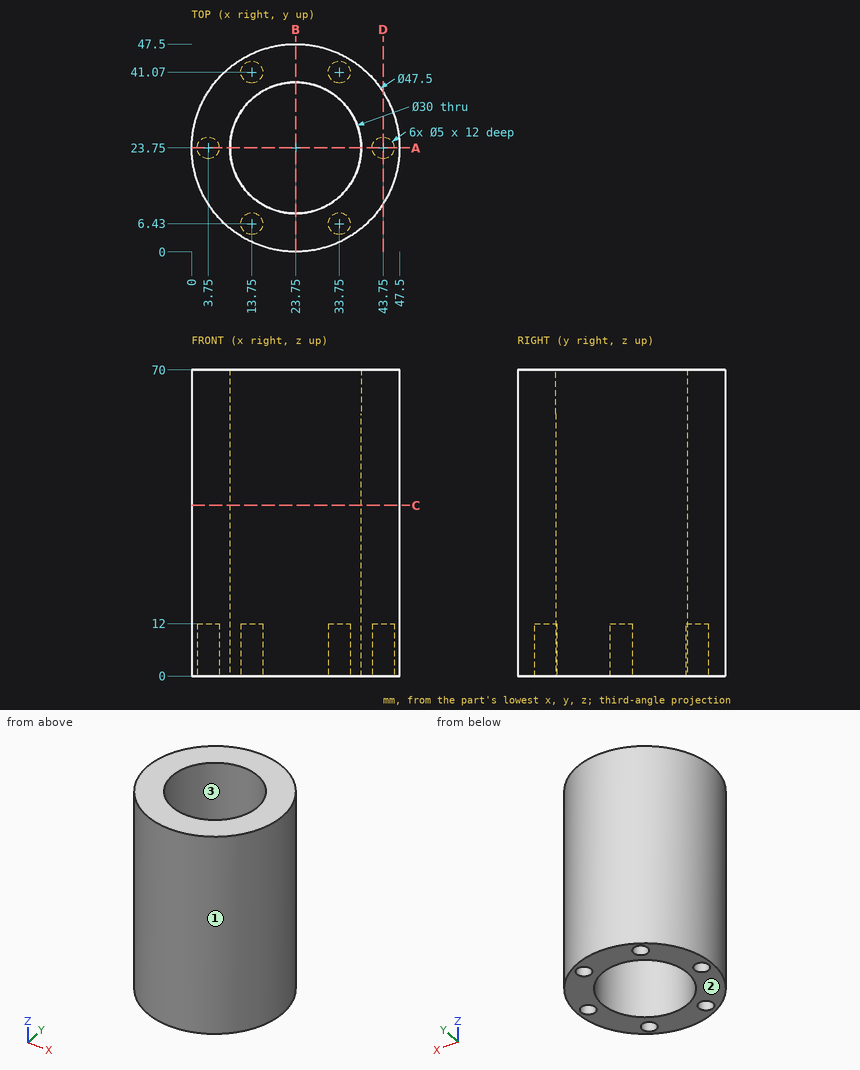
Could you check a few things on this drawing? It's one solid part, dimensions in mm from its lowest x, y, z. Round coordinates to 2 decimals unless told otherwise and drop trailing zeros. Write each loop counter-clockwise with the first axis right and the second up, starting at its lowest first coordinate (ties: lowest second). Pieces come first, ordered by that corner, then holes. Notation, with made-up numbers: (14.5, -23.5) -> (37.5, -23.5) arc R14 cw to (37.5, -13.5) -> close; hole circle Ø9 at (45, 84). An arc over 180 degrees is marked (long way). One line per item, written item: value.
1) We'd pull the mould along Y, two halves only. Please class the marked faces 1, 2 and 3: released by +Y, released by -Y, zero draft, split by the parting line, or undercut.
Filled sheet:
face 1: split by the parting line
face 2: zero draft
face 3: undercut
2) If I drill on line 1 (X direction, y = 23.75, z = 3.5); line 2 (Y direction, x = 33, z = 3) (1 decimal); line 3 (Y direction, x = 23.5, z = 34.5), over which ranges is the centre line in solid material (lowest first)? Write a range as [from, to].
Filled sheet:
line 1: x = [0, 1.25], [6.25, 8.75], [38.75, 41.25], [46.25, 47.5]
line 2: y = [1.9, 4], [8.8, 11.9], [35.6, 38.7], [43.5, 45.6]
line 3: y = [0, 8.75], [38.75, 47.5]
3) Suppose I cut it at A-A on y = 23.75. List the corners of the cut face in (x, z) for me.
Filled sheet:
outline: (0, 0) -> (1.25, 0) -> (1.25, 12) -> (6.25, 12) -> (6.25, 0) -> (8.75, 0) -> (8.75, 70) -> (0, 70) -> close; (38.75, 0) -> (41.25, 0) -> (41.25, 12) -> (46.25, 12) -> (46.25, 0) -> (47.5, 0) -> (47.5, 70) -> (38.75, 70) -> close
4) Suppose I cut it at D-D on x = 43.75. List the corners of the cut face in (y, z) for me, plus the area to 3 significant figures.
Filled sheet:
outline: (10.94, 0) -> (21.25, 0) -> (21.25, 12) -> (26.25, 12) -> (26.25, 0) -> (36.56, 0) -> (36.56, 70) -> (10.94, 70) -> close
area: 1,730 mm2
5) I'm going to push flat-ended pins straight in: pin 1 Ø5 at (x, z) = (7, 49) entering from -Y; pin 2 Ø4.5 at (x, y) = (33.75, 41.07) entering from -Z; pin 3 Ø4 at (x, z) = (8.5, 25.5) entering from +Y. Where does each tip first touch, or does it pass through?
Filled sheet:
pin 1: stops at y = 4.75
pin 2: stops at z = 12
pin 3: stops at y = 43.46
6) Suppose I cut it at C-C on z = 39. List the corners of the cut face in (x, y) for me.
Filled sheet:
outline: circle Ø47.5 at (23.75, 23.75); hole circle Ø30 at (23.75, 23.75)
7) Suppose I cut it at B-B on x = 23.75. List the corners of the cut face in (y, z) for me, plus the area to 4 significant figures.
Filled sheet:
outline: (0, 0) -> (8.75, 0) -> (8.75, 70) -> (0, 70) -> close; (38.75, 0) -> (47.5, 0) -> (47.5, 70) -> (38.75, 70) -> close
area: 1,225 mm2
